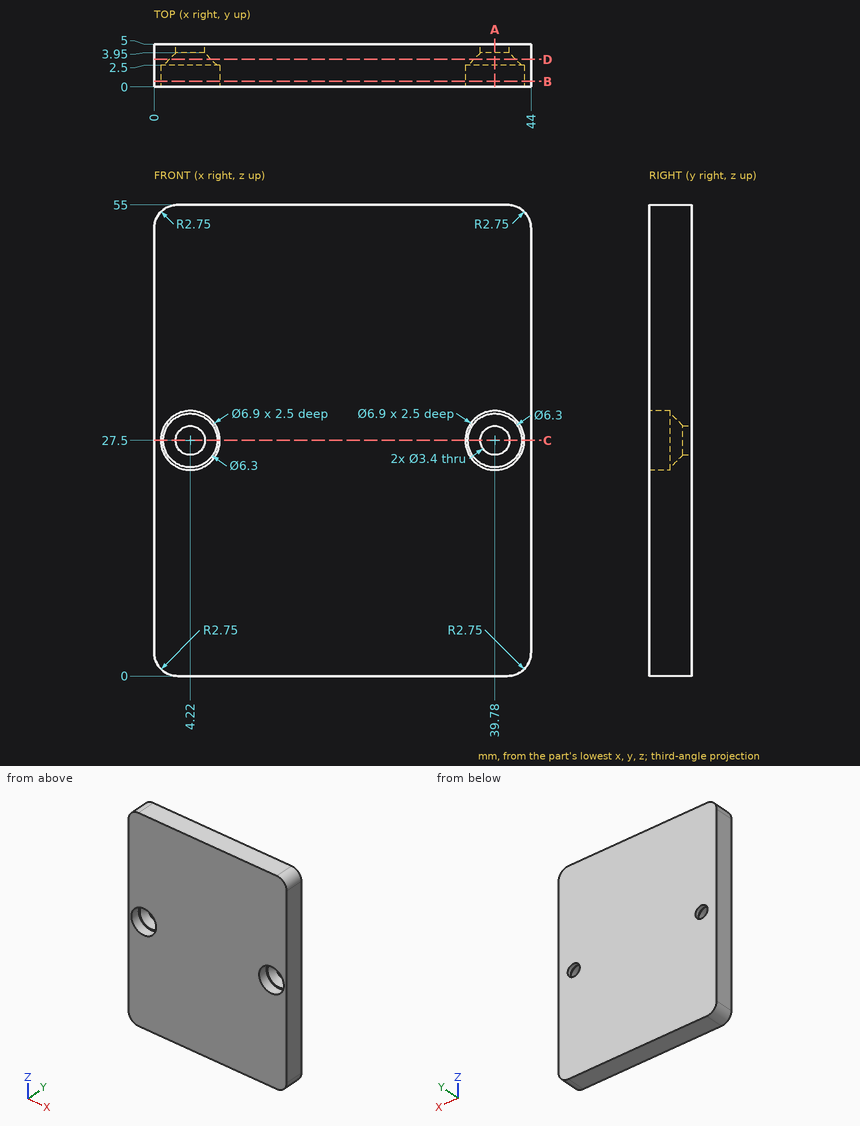
Here's the drawing with two shaded views (mm, measured from the low corner). I have some questions. Give positions to 0.01 mm unless a question says otherwise; leave off trailing zeros. Write each loop counter-clockwise with the first axis right and the second up, starting at its lowest first coordinate (ties: lowest second). Pieces come first, ordered by that corner, then holes. Notation, with made-up numbers: (-15, 36) -> (36, 36) arc R30 ccw to (36, 74) -> close; hole circle Ø7 at (-34, 46.5). An arc over 180 degrees is marked (long way). One line per item, written item: value.
Q1. Imagine slicing it at B-B on y = 0.65. Please give me the cut outline in (x, z), and give its area (3 significant figures).
Results found:
outline: (0, 2.75) arc R2.75 ccw to (2.75, 0) -> (41.25, 0) arc R2.75 ccw to (44, 2.75) -> (44, 52.25) arc R2.75 ccw to (41.25, 55) -> (2.75, 55) arc R2.75 ccw to (0, 52.25) -> close; hole circle Ø6.9 at (4.22, 27.5); hole circle Ø6.9 at (39.78, 27.5)
area: 2,340 mm^2
Q2. For P1, Ø6, axis at x = 39.78, z = 27.5, coming from the -Y side; P2, Ø4, axis at x = 39.78, z = 27.5, coming from the -Y side; P3, Ø4.5, axis at x = 4.22, z = 27.5, coming from the -Y side, each with a flat end and sliding along its axis, tell me the tip position at first contact or that it passes through.
Results found:
P1: stops at y = 2.65
P2: stops at y = 3.65
P3: stops at y = 3.4
Q3. Please list where these lines run through material, in increasing order: line 1 (X direction, y = 1.8, z = 27.5); line 2 (X direction, y = 4.4, z = 27.5); line 3 (Z direction, x = 39, y = 0.5). Write a range as [from, to].
Results found:
line 1: x = [0, 0.77], [7.67, 36.33], [43.23, 44]
line 2: x = [0, 2.52], [5.92, 38.08], [41.48, 44]
line 3: z = [0, 24.14], [30.86, 55]
Q4. Imagine slicing it at C-C on z = 27.5. Please give me the cut outline in (x, y).
Results found:
outline: (0, 0) -> (0.77, 0) -> (0.77, 2.5) -> (1.07, 2.5) -> (2.52, 3.95) -> (2.52, 5) -> (0, 5) -> close; (5.92, 3.95) -> (7.37, 2.5) -> (7.67, 2.5) -> (7.67, 0) -> (36.33, 0) -> (36.33, 2.5) -> (36.63, 2.5) -> (38.08, 3.95) -> (38.08, 5) -> (5.92, 5) -> close; (41.48, 3.95) -> (42.93, 2.5) -> (43.23, 2.5) -> (43.23, 0) -> (44, 0) -> (44, 5) -> (41.48, 5) -> close
Q5. Imagine slicing it at A-A on x = 39.78. Please give me the cut outline in (y, z), and give its area (3 significant figures).
Results found:
outline: (0, 0) -> (5, 0) -> (5, 25.8) -> (3.95, 25.8) -> (2.5, 24.35) -> (2.5, 24.05) -> (0, 24.05) -> close; (0, 30.95) -> (2.5, 30.95) -> (2.5, 30.65) -> (3.95, 29.2) -> (5, 29.2) -> (5, 55) -> (0, 55) -> close
area: 247 mm^2
Q6. Imagine slicing it at D-D on y = 3.2. Please give me the cut outline in (x, z), and give its area (3 significant figures).
Results found:
outline: (0, 2.75) arc R2.75 ccw to (2.75, 0) -> (41.25, 0) arc R2.75 ccw to (44, 2.75) -> (44, 52.25) arc R2.75 ccw to (41.25, 55) -> (2.75, 55) arc R2.75 ccw to (0, 52.25) -> close; hole circle Ø4.9 at (4.22, 27.5); hole circle Ø4.9 at (39.78, 27.5)
area: 2,380 mm^2
